```python
from build123d import *

# Parameters (mm, degrees)
SKETCH1_W           = 40
SKETCH1_H           = 40
BOSS_EXTRUDE1_DEPTH = 40
SKETCH2_W           = 5
SKETCH2_H           = 20
CUT_EXTRUDE1_DEPTH  = 40
CUT_EXTRUDE2_DEPTH  = 40
SKETCH4_W           = 10
SKETCH4_H           = 30
CUT_EXTRUDE3_DEPTH  = 40
SKETCH5_W           = 30
SKETCH5_H           = 20
CUT_EXTRUDE4_DEPTH  = 40


with BuildPart() as part:
    # Sketch1 → Boss-Extrude1 (new body)
    with BuildSketch(Plane.XY):
        with Locations((20, 20)):
            Rectangle(SKETCH1_W, SKETCH1_H)
    extrude(amount=BOSS_EXTRUDE1_DEPTH)

    # Sketch2 → Cut-Extrude1 (cut)
    with BuildSketch(Plane.XY.offset(40)):
        with Locations((2.5, 30)):
            Rectangle(SKETCH2_W, SKETCH2_H)
    extrude(amount=-CUT_EXTRUDE1_DEPTH, mode=Mode.SUBTRACT)

    # Sketch3 → Cut-Extrude2 (cut)
    with BuildSketch(Plane(origin=(0, 0, 0), x_dir=(1, 0, 0), z_dir=(0, 1, 0))):
        with BuildLine():
            ThreePointArc((0, -20.000000105), (5.857864339, -5.857864414), (20, 0))
            Line((20, 0), (0, 0))
            Line((0, 0), (0, -20.000000105))
        make_face()
        with BuildLine():
            ThreePointArc((20, -40), (5.857864414, -34.142135661), (0, -20.000000105))
            Line((0, -20.000000105), (0, -40))
            Line((0, -40), (20, -40))
        make_face()
    extrude(amount=CUT_EXTRUDE2_DEPTH, mode=Mode.SUBTRACT)

    # Sketch4 → Cut-Extrude3 (cut)
    with BuildSketch(Plane(origin=(0, 40, 0), x_dir=(1, 0, 0), z_dir=(0, 1, 0))):
        with Locations((35, -25)):
            Rectangle(SKETCH4_W, SKETCH4_H)
    extrude(amount=-CUT_EXTRUDE3_DEPTH, mode=Mode.SUBTRACT)

    # Sketch5 → Cut-Extrude4 (cut)
    with BuildSketch(Plane(origin=(30, 0, 0), x_dir=(0, 0, -1), z_dir=(1, 0, 0))):
        with Locations((-25, 30)):
            Rectangle(SKETCH5_W, SKETCH5_H)
    extrude(amount=-CUT_EXTRUDE4_DEPTH, mode=Mode.SUBTRACT)


solid = part.part
```
Geometry: final body of the model. Coordinates: model frame, mm. A direction names the side the tool comes from. Coordinates: 2 decimals unless noted, no trailing zeros. Order: outer loops, then holes, each group sorted by start corner. A loop starts at its lowest first (then second) coordinate and runs counter-clockwise, first axis right, second up. Notation, with made-up numbers: (74, -33.75) - (133, -33.75) arc R9 cw to (133, -21.75) - close; hole circle Ø11 at (-5, 89.5). An arc over 180 degrees is marked (long way). Return JSON: item names as keys, results as strings. Group by question number.
1. Pin query (flat end, axial travel): pin 1 (16 mm diameter, centred on y = 8.5, z = 26.5, fed in from +X); pin 2 (8 mm diameter, centred on y = 6.5, z = 6, fed in from -X); pin 3 (1.6 mm diameter, centred on y = 35, z = 8.5, fed in from -X). Return the tip coordinate at first contact, or that it passes through.
2. Material intervals for line 1 along Y through (x, z) = (21, 30.5); line 2 along Z through (x, y) = (37.5, 20.5); line 3 along X through (y, z) = (24.5, 7), sorted ascending. Write a range as [from, to].
3. Set-up query: faces 1 (the face through (5, 30, 8)), 2 (the face through (20, 0, 20)), 3 (the face through (30, 10, 25)). Return all of +Z, -Z, +X, -X, +Y, -Y with unobstructed straight access to the full face (end or side cutting, diameter ignored); none if empty.
4. Cut plane C-C (z = 32). Output: boundary loops of the cut face in (x, y).
5. Cut plane B-B (x = 25). Output: boundary loops of the cut face in (y, z).
6. Cut plane A-A (y = 19). Output: boundary loops of the cut face in (x, z), plus the area to 3 significant figures.
7. Cut plane D-D (z = 5). Output: boundary loops of the cut face in (x, y), plus the area to 3 significant figures.
Resolved:
{
 "1": {"pin 1": "stops at x = 30", "pin 2": "stops at x = 2.68", "pin 3": "stops at x = 5"},
 "2": {"line 1": "y = [0, 20]", "line 2": "z = [0, 10]", "line 3": "x = [5, 40]"},
 "3": {"face 1": "+Z, -Z, -X, +Y", "face 2": "+Z, -Z, +X, -X, -Y", "face 3": "+Z, +X, +Y, -Y"},
 "4": {"outline": "(4, 0) - (30, 0) - (30, 20) - (4, 20) - close"},
 "5": {"outline": "(0, 0) - (40, 0) - (40, 10) - (20, 10) - (20, 40) - (0, 40) - close"},
 "6": {"outline": "(20, 0) - (40, 0) - (40, 10) - (30, 10) - (30, 40) - (20, 40) arc R20 ccw to start", "area": "1,130 mm²"},
 "7": {"outline": "(6.77, 0) - (40, 0) - (40, 40) - (6.77, 40) - close", "area": "1,330 mm²"}
}
